For this review, take the finished solid that the model builds, in its own axes (mm). Round coordinates to 2 decimals unless told otherwise and drop trailing zeros. Loops run counter-clockwise (first coordinate to the right, second up) from the corner with the lowest first, then second, coordinate; pieces in that order, holes last.
1) Take a section at C-C (z = -4.75). State the section outline as (x, y) points, then the cut area to 3 significant figures.
2) Take a section at B-B (x = 0). State the section outline as (y, z) points.
3) Wall thickness on L1, parallel to Y at x = 0, z = -1; L2, parallel to Y at x = 0.5, z = 5.25; L3, parallel to X at y = 1.5, z = 4.75: over which ranges is each line inside the solid? List them lowest first.
4) Mouldability with a two-part tool opening along Y and no side actions: class faces 1 (the flat face through (-2, -1, 6)), 2 (the cylindrical face through (0, -2, 0)), 3 (the flat face through (0, -5.444, 0)) as pulls with the +Y half, pulls with the -Y half, needs draft (parallel to the pull), parting line crosses it, or undercut.
5) Take a section at A-A (y = 0). State the section outline as (x, z) points.
```python
from build123d import *

# Parameters (mm, degrees)
F0_R          = 19.05
F0_R_2        = 7.9375
F1_DEPTH      = 25.4
F3_W          = 16.0429216921
F3_H          = 10.8887040988
F3_R          = 2
F4_DEPTH      = 6
F4_DEPTH_BACK = 6


# Not quite as in the source:
# - the program builds the solid bodies; features that only make, move or delete a surface that nothing else refers to are left out


with BuildPart() as f1:
    # F0 (on Top) → F1 (new body)
    with BuildSketch(Plane.XY):
        Circle(F0_R)
        Circle(F0_R_2, mode=Mode.SUBTRACT)
    extrude(amount=F1_DEPTH)


with BuildPart() as f4:
    # F3 (on Top) → F4 (new body, two sides)
    with BuildSketch(Plane.XY) as f4_sk:
        Rectangle(F3_W, F3_H)
        Circle(F3_R, mode=Mode.SUBTRACT)
    extrude(amount=F4_DEPTH)
    extrude(f4_sk.sketch, amount=-F4_DEPTH_BACK)


solid = f4.part
```
Response:
1. outline: (-8.02, -5.44) - (8.02, -5.44) - (8.02, 5.44) - (-8.02, 5.44) - close; hole circle Ø4 at (0, 0)
1. area: 162 mm2
2. outline: (-5.44, -6) - (-2, -6) - (-2, 6) - (-5.44, 6) - close; (2, -6) - (5.44, -6) - (5.44, 6) - (2, 6) - close
3. L1: y = -5.44 to -2, 2 to 5.44
3. L2: y = -5.44 to -1.94, 1.94 to 5.44
3. L3: x = -8.02 to -1.32, 1.32 to 8.02
4. face 1: needs draft
4. face 2: undercut
4. face 3: pulls with the -Y half
5. outline: (-8.02, -6) - (-2, -6) - (-2, 6) - (-8.02, 6) - close; (2, -6) - (8.02, -6) - (8.02, 6) - (2, 6) - close
